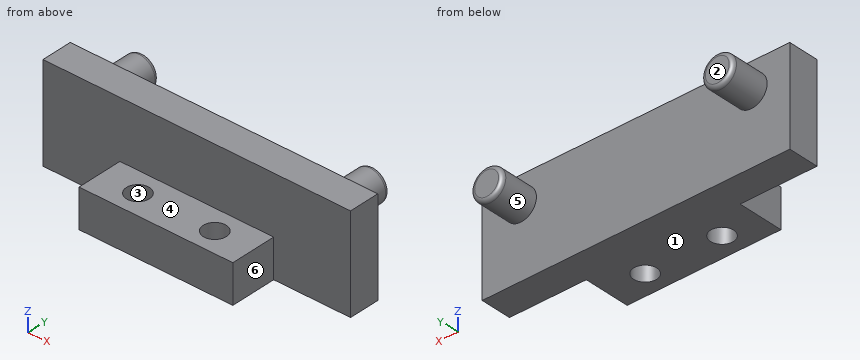
```python
from build123d import *

# Parameters (mm, degrees)
SKETCH_1_W      = 20
SKETCH_1_H      = 10
SKETCH_1_R      = 1.5
EXTRUDE_1_DEPTH = 5
SKETCH_2_W      = 40
SKETCH_2_H      = 12.5
EXTRUDE_2_DEPTH = 4
SKETCH_3_R      = 2.05
EXTRUDE_3_DEPTH = 5
FILLET_1_R      = 0.5


with BuildPart() as part:
    # 草图1 → 凸台-拉伸1 (new body)
    with BuildSketch(Plane.XY):
        with Locations((0, 5)):
            Rectangle(SKETCH_1_W, SKETCH_1_H)
        with Locations((-5, 3)):
            Circle(SKETCH_1_R, mode=Mode.SUBTRACT)
        with Locations((5, 3)):
            Circle(SKETCH_1_R, mode=Mode.SUBTRACT)
    extrude(amount=EXTRUDE_1_DEPTH)

    # 草图2 → 凸台-拉伸2 (add)
    with BuildSketch(Plane(origin=(0, 10, 0), x_dir=(1, 0, 0), z_dir=(0, 1, 0))):
        with Locations((0, -6.25)):
            Rectangle(SKETCH_2_W, SKETCH_2_H)
    extrude(amount=-EXTRUDE_2_DEPTH)

    # 草图3 → 凸台-拉伸3 (add)
    with BuildSketch(Plane(origin=(0, 10, 0), x_dir=(1, 0, 0), z_dir=(0, 1, 0))):
        with Locations((-15, -9)):
            Circle(SKETCH_3_R)
        with Locations((15, -9)):
            Circle(SKETCH_3_R)
    extrude(amount=EXTRUDE_3_DEPTH)

    # 圆角1
    fillet_1_edges = [part.edges().sort_by_distance(p)[0] for p in [
        (-17.05, 15, 9),
        (12.95, 15, 9),
    ]]
    fillet(fillet_1_edges, radius=FILLET_1_R)


solid = part.part
```
Verification items for the finished model (mm, model axes). Face numbers are marked on the shaded views. A direction names the side the tool comes from. Round coordinates to 2 decimals unless told otherwise and drop trailing zeros. Order: outer loops, then holes, each group sorted by start corner. A loop starts at its lowest first (then second) coordinate and runs counter-clockwise, first axis right, second up.
1) Material ranges on line 1 (Y direction, x = -5, z = 3.35); line 2 (Y direction, x = 7, z = 5.25); line 3 (Y direction, x = 0.5, z = 4), recorded low to high.
Geometry says:
line 1: y = 0 to 1.5, 4.5 to 10
line 2: y = 6 to 10
line 3: y = 0 to 10
2) Tool access check on the marked faces 4, 5 and 6. Record the directions out of +Z, -Z, +X, -X, +Y, -Y that give a thin tool (end or side, any length) a straight path to the whole face; none if there is none.
Geometry says:
face 4: +Z, +X, -X, -Y
face 5: +Y
face 6: +Z, -Z, +X, -Y
3) Cross-section at A-A, the plane z = 4. Record the cut outline in (x, y).
Geometry says:
outline: (-20, 6) - (-10, 6) - (-10, 0) - (10, 0) - (10, 6) - (20, 6) - (20, 10) - (-20, 10) - close; hole circle Ø3 at (-5, 3); hole circle Ø3 at (5, 3)
4) Depth check by flat-ended pin: pin 1 (1.8 mm diameter, centred on x = 5, y = 3, fed in from -Z); pin 2 (6 mm diameter, centred on x = 6.5, z = 8, fed in from +Y); pin 3 (1.8 mm diameter, centred on x = -4, y = 3.5, fed in from +Z); pin 4 (5 mm diameter, centred on y = 5.5, z = 4.5, fed in from +X). Enter the tip coordinate at first touch or a pass-through.
Geometry says:
pin 1: passes through
pin 2: stops at y = 10
pin 3: stops at z = 5
pin 4: stops at x = 20
5) Cross-section at C-C, the plane x = 15. Record the cut outline in (y, z).
Geometry says:
outline: (6, 0) - (10, 0) - (10, 6.95) - (14.5, 6.95) arc R0.5 ccw to (15, 7.45) - (15, 10.55) arc R0.5 ccw to (14.5, 11.05) - (10, 11.05) - (10, 12.5) - (6, 12.5) - close
6) Cross-section at B-B, the plane x = -5. Record the cut outline in (y, z).
Geometry says:
outline: (0, 0) - (1.5, 0) - (1.5, 5) - (0, 5) - close; (4.5, 0) - (10, 0) - (10, 12.5) - (6, 12.5) - (6, 5) - (4.5, 5) - close
7) Draft check along Y on the marked faces 1, 2 and 3. Enter one of: +Y half, -Y half, draft (parallel to the pull), parting line (faces both ways), or undercut.
Geometry says:
face 1: draft
face 2: +Y half
face 3: undercut
